Here's how the part is built. I have some questions about the finished solid (model axes, mm). A direction names the side the tool comes from. Coordinates: 2 decimals unless noted, no trailing zeros. Write each loop counter-clockwise with the first axis right and the second up, starting at its lowest first coordinate (ties: lowest second). Pieces come first, ordered by that corner, then holes. Notation, with made-up numbers: (-18.5, -9) -> (33.5, -9) arc R9 cw to (33.5, 4) -> close; hole circle Ø11 at (63.5, -28.75). An arc over 180 degrees is marked (long way). Use a Markdown table: item, result. Add a question column.
Item 1: Imagine slicing it at A-A, the plane x = 87. Write out the boundary of the cut face in (y, z).
Item 2: Will these pins go through, and if not, where does the flat tip stop? pin 1 Ø2.5 at (x, y) = (93.5, 45.5) entering from -Z; pin 2 Ø1.5 at (y, z) = (45.5, 1) entering from +X; pin 3 Ø7 at (x, y) = (-116, 28.18) entering from -Z.
Item 3: Imagine slicing it at B-B, the plane y = -3. Write out the boundary of the cut face in (x, z), and give its area (3 significant figures).
Item 4: If we mould it in two halves opening along X, with no side actions, what happens to faces 3 (the cylindrical face through (-66.77, 13.35, 1.52)), 4 (the flat face through (-134, -3, 1)), 5 (the flat face through (157, 87, 2))? For each: pulls with the +X half, pulls with the -X half, needs draft (parallel to the pull), parting line crosses it, or undercut.
Item 5: If I drill on line 1 along X through (y, z) = (32, 0.8); line 2 along Y through (x, z) = (115.25, 2.15); line 3 along Y through (x, z) = (-4, 0.8), over which ranges is the centre line in solid material (lowest first)? Write a range as from..to.
Item 6: On a 3-axis mill with a long thin cutter (end or side, diameter ignored), from which of +Z, -Z, +X, -X, +Y, -Y can I reach the whole of each face in a straight line? I mean faces 1 (the flat face through (16.99, 89.02, 1.52)), 2 (the flat face through (13, 59, 3)). Say none if no direction works.
Item 7: Imagine slicing it at C-C, the plane z = 1.2. Count the separate pieces of the cut face and the enclosed holes in it, and give its area (3 significant figures).
```python
from build123d import *

# Parameters (mm, degrees)
SKETCH1_W           = 274
SKETCH1_H           = 44
BOSS_EXTRUDE1_DEPTH = 3
SKETCH2_W           = 3
SKETCH2_H           = 25
CUT_EXTRUDE1_DEPTH  = 144.923590839
SKETCH3_W           = 274
SKETCH3_H           = 6
BOSS_EXTRUDE2_DEPTH = 3
SKETCH4_W           = 80
SKETCH4_H           = 3
CUT_EXTRUDE2_DEPTH  = 146.869804963
SKETCH6_R           = 2.1
CUT_EXTRUDE3_DEPTH  = 146.869804963
CUT_EXTRUDE4_DEPTH  = 146.869804963
SKETCH8_R           = 1.5
CUT_EXTRUDE5_DEPTH  = 3
BOSS_EXTRUDE4_DEPTH = 3
BOSS_EXTRUDE5_DEPTH = 3
FILLET2_R           = 5
BOSS_EXTRUDE6_DEPTH = 3
FILLET3_R           = 2
SKETCH13_W          = 3
SKETCH13_H          = 15
CUT_EXTRUDE6_DEPTH  = 3
CHAMFER2_SIZE       = 10
FILLET4_R           = 2
FILLET5_R           = 5
CUT_EXTRUDE9_DEPTH  = 220.631509579
FILLET6_R           = 5.5
BOSS_EXTRUDE7_DEPTH = 3
FILLET7_R           = 10
SKETCH18_R          = 4.1
CUT_EXTRUDE10_DEPTH = 220.631509579
SKETCH19_R          = 1.6
SKETCH19_W          = 3
SKETCH19_H          = 25
CUT_EXTRUDE11_DEPTH = 220.631509579
SKETCH20_R          = 3.1
CUT_EXTRUDE12_DEPTH = 220.631509579
SKETCH21_R          = 0.8
CUT_EXTRUDE13_DEPTH = 220.631509579
SKETCH22_R          = 2.1
CUT_EXTRUDE14_DEPTH = 220.631509579
SKETCH23_W          = 50
SKETCH23_H          = 25
CUT_EXTRUDE15_DEPTH = 220.631509579
FILLET8_R           = 3
SKETCH25_R          = 2.1
CUT_EXTRUDE16_DEPTH = 220.631509579


with BuildPart() as part:
    # Sketch1 → Boss-Extrude1 (new body)
    with BuildSketch(Plane.XY):
        with Locations((0, 22)):
            Rectangle(SKETCH1_W, SKETCH1_H)
    extrude(amount=BOSS_EXTRUDE1_DEPTH)

    # Sketch2 → Cut-Extrude1 (cut, through all)
    with BuildSketch(Plane.XY.offset(3)):
        with Locations((-93.5, 22)):
            Rectangle(SKETCH2_W, SKETCH2_H)
        with Locations((93.5, 22)):
            Rectangle(SKETCH2_W, SKETCH2_H)
    extrude(amount=-CUT_EXTRUDE1_DEPTH, mode=Mode.SUBTRACT)

    # Sketch3 → Boss-Extrude2 (add)
    with BuildSketch(Plane.XY.offset(3)):
        with Locations((0, 47)):
            Rectangle(SKETCH3_W, SKETCH3_H)
    extrude(amount=-BOSS_EXTRUDE2_DEPTH)

    # Sketch4 → Cut-Extrude2 (cut, through all)
    with BuildSketch(Plane.XY.offset(3)):
        with Locations((0, 45.5)):
            Rectangle(SKETCH4_W, SKETCH4_H)
    extrude(amount=-CUT_EXTRUDE2_DEPTH, mode=Mode.SUBTRACT)

    # Sketch6 → Cut-Extrude3 (cut, through all)
    with BuildSketch(Plane(origin=(0, 0, 0), x_dir=(-1, 0, 0), z_dir=(0, 0, -1))):
        with Locations((62.874847501, 21)):
            Circle(SKETCH6_R)
    extrude(amount=-CUT_EXTRUDE3_DEPTH, mode=Mode.SUBTRACT)

    # Sketch7 → Cut-Extrude4 (cut, through all)
    with BuildSketch(Plane(origin=(0, 0, 0), x_dir=(-1, 0, 0), z_dir=(0, 0, -1))):
        Polygon((0, 15), (-68.339745962, 15), (-77, 0), (0, 0), align=None)
        Polygon((68.339745962, 15), (0, 15), (0, 0), (77, 0), align=None)
    extrude(amount=-CUT_EXTRUDE4_DEPTH, mode=Mode.SUBTRACT)

    # Sketch8 → Cut-Extrude5 (cut)
    with BuildSketch(Plane(origin=(0, 0, 0), x_dir=(-1, 0, 0), z_dir=(0, 0, -1))):
        with Locations((-93.5, 45.5)):
            Circle(SKETCH8_R)
        with Locations((-115.25, 4.75)):
            Circle(SKETCH8_R)
        with Locations((-71.75, 4.75)):
            Circle(SKETCH8_R)
        with Locations((71.75, 4.75)):
            Circle(SKETCH8_R)
        with Locations(Location((115.25, 4.75, 0), (0, 0, 180))):
            Circle(SKETCH8_R)
        with Locations(Location((93.5, 45.5, 0), (0, 0, 180))):
            Circle(SKETCH8_R)
    extrude(amount=-CUT_EXTRUDE5_DEPTH, mode=Mode.SUBTRACT)

    # Sketch9 → Boss-Extrude4 (add)
    with BuildSketch(Plane(origin=(0, 0, 0), x_dir=(-1, 0, 0), z_dir=(0, 0, -1))):
        Polygon((137, 0), (122, -15), (68.339745962, -15), (68.339745962, 15), (77, 0), align=None)
    extrude(amount=-BOSS_EXTRUDE4_DEPTH)

    # Sketch10 → Boss-Extrude5 (add)
    with BuildSketch(Plane.XY.offset(3)):
        Polygon((137, 50), (137, 130), (72, 130), (72, 126.069778962), (-137, 50), align=None)
        Polygon((-51.754445725, 64), (67, 107.223083431), (67, 64), align=None, mode=Mode.SUBTRACT)
    extrude(amount=-BOSS_EXTRUDE5_DEPTH)

    # Fillet2
    fillet2_edges = [part.edges().sort_by_distance(p)[0] for p in [
        (67, 64, 1.5),
        (67, 107.223083431, 1.5),
        (-51.754445725, 64, 1.5),
    ]]
    fillet(fillet2_edges, radius=FILLET2_R)

    # Sketch11 → Boss-Extrude6 (add)
    with BuildSketch(Plane.XY.offset(3)):
        Polygon((137, 44), (154.942501021, 44), (137, 82.576377194), (137, 130), (177, 44), (177, 0), (137, 0), align=None)
    extrude(amount=-BOSS_EXTRUDE6_DEPTH)

    # Fillet3
    fillet3_edges = [part.edges().sort_by_distance(p)[0] for p in [
        (137, 44, 1.5),
        (154.942501021, 44, 1.5),
        (137, 82.576377194, 1.5),
    ]]
    fillet(fillet3_edges, radius=FILLET3_R)

    # Sketch13 → Cut-Extrude6 (cut)
    with BuildSketch(Plane.XY.offset(3)):
        with Locations((167.5, 22)):
            Rectangle(SKETCH13_W, SKETCH13_H)
    extrude(amount=-CUT_EXTRUDE6_DEPTH, mode=Mode.SUBTRACT)

    # Chamfer2
    chamfer2_edges = [part.edges().sort_by_distance(p)[0] for p in [
        (177, 0, 1.5),
    ]]
    chamfer(chamfer2_edges, length=CHAMFER2_SIZE)

    # Fillet4
    fillet4_edges = [part.edges().sort_by_distance(p)[0] for p in [
        (137, 130, 1.5),
        (72, 130, 1.5),
        (72, 126.069778962, 1.5),
        (177, 44, 1.5),
    ]]
    fillet(fillet4_edges, radius=FILLET4_R)

    # Fillet5
    fillet5_edges = [part.edges().sort_by_distance(p)[0] for p in [
        (-68.339745962, -15, 1.5),
        (-122, -15, 1.5),
        (167, 0, 1.5),
        (177, 10, 1.5),
        (77, 0, 1.5),
    ]]
    fillet(fillet5_edges, radius=FILLET5_R)

    # Sketch15 → Cut-Extrude9 (cut, through all)
    with BuildSketch(Plane(origin=(0, 0, 0), x_dir=(-1, 0, 0), z_dir=(0, 0, -1))):
        Polygon((-68.339745962, 15), (-61.411542732, 27), (54.936767243, 27), (58.339745962, 15), align=None)
    extrude(amount=-CUT_EXTRUDE9_DEPTH, mode=Mode.SUBTRACT)

    # Fillet6
    fillet6_edges = [part.edges().sort_by_distance(p)[0] for p in [
        (-58.339745962, 15, 1.5),
        (61.411542732, 27, 1.5),
        (-54.936767243, 27, 1.5),
        (-68.339745962, 15, 1.5),
    ]]
    fillet(fillet6_edges, radius=FILLET6_R)

    # Sketch17 → Boss-Extrude7 (add)
    with BuildSketch(Plane(origin=(0, 0, 0), x_dir=(-1, 0, 0), z_dir=(0, 0, -1))):
        Polygon((137, 50), (147, 46.360297657), (147, 10), (137, 0), align=None)
    extrude(amount=-BOSS_EXTRUDE7_DEPTH)

    # Fillet7
    fillet7_edges = [part.edges().sort_by_distance(p)[0] for p in [
        (-147, 10, 1.5),
        (-147, 46.360297657, 1.5),
    ]]
    fillet(fillet7_edges, radius=FILLET7_R)

    # Sketch18 → Cut-Extrude10 (cut, through all)
    with BuildSketch(Plane.XY.offset(3)):
        with Locations((87, 117)):
            Circle(SKETCH18_R)
        with Locations((127, 117)):
            Circle(SKETCH18_R)
        with Locations((87, 87.509284164)):
            Circle(SKETCH18_R)
        with Locations((127, 87.509284164)):
            Circle(SKETCH18_R)
    extrude(amount=-CUT_EXTRUDE10_DEPTH, mode=Mode.SUBTRACT)

    # Sketch19 → Cut-Extrude11 (cut, through all)
    with BuildSketch(Plane.XY.offset(3)):
        with Locations((128.5, 45.5)):
            Circle(SKETCH19_R)
        with Locations((128.5, 22)):
            Rectangle(SKETCH19_W, SKETCH19_H)
    extrude(amount=-CUT_EXTRUDE11_DEPTH, mode=Mode.SUBTRACT)

    # Sketch20 → Cut-Extrude12 (cut, through all)
    with BuildSketch(Plane(origin=(0, 0, 0), x_dir=(-1, 0, 0), z_dir=(0, 0, -1))):
        with Locations((116, 28.180148829)):
            Circle(SKETCH20_R)
    extrude(amount=-CUT_EXTRUDE12_DEPTH, mode=Mode.SUBTRACT)

    # Sketch21 → Cut-Extrude13 (cut, through all)
    with BuildSketch(Plane(origin=(0, 0, 0), x_dir=(-1, 0, 0), z_dir=(0, 0, -1))):
        with Locations((-166, 28.7)):
            Circle(SKETCH21_R)
        with Locations((-169, 15.3)):
            Circle(SKETCH21_R)
        with Locations((-166, 15.3)):
            Circle(SKETCH21_R)
        with Locations((-130, 33.7)):
            Circle(SKETCH21_R)
        with Locations((-127, 33.7)):
            Circle(SKETCH21_R)
        with Locations((-130, 10.3)):
            Circle(SKETCH21_R)
        with Locations((-127, 10.3)):
            Circle(SKETCH21_R)
        with Locations((-95, 33.7)):
            Circle(SKETCH21_R)
        with Locations((-92, 33.7)):
            Circle(SKETCH21_R)
        with Locations((-95, 10.3)):
            Circle(SKETCH21_R)
        with Locations((-92, 10.3)):
            Circle(SKETCH21_R)
        with Locations((-40, 47)):
            Circle(SKETCH21_R)
        with Locations((-40, 44)):
            Circle(SKETCH21_R)
        with Locations((40, 47)):
            Circle(SKETCH21_R)
        with Locations((40, 44)):
            Circle(SKETCH21_R)
        with Locations((95, 33.7)):
            Circle(SKETCH21_R)
        with Locations((95, 10.3)):
            Circle(SKETCH21_R)
        with Locations((-169, 28.7)):
            Circle(SKETCH21_R)
        with Locations((92, 33.7)):
            Circle(SKETCH21_R)
        with Locations((92, 10.3)):
            Circle(SKETCH21_R)
    extrude(amount=-CUT_EXTRUDE13_DEPTH, mode=Mode.SUBTRACT)

    # Sketch22 → Cut-Extrude14 (cut, through all)
    with BuildSketch(Plane(origin=(0, 0, 0), x_dir=(-1, 0, 0), z_dir=(0, 0, -1))):
        with Locations((0, 51)):
            Circle(SKETCH22_R)
        with Locations((-25, 51)):
            Circle(SKETCH22_R)
        with Locations(Location((25, 51, 0), (0, 0, 180))):
            Circle(SKETCH22_R)
    extrude(amount=-CUT_EXTRUDE14_DEPTH, mode=Mode.SUBTRACT)

    # Sketch23 → Cut-Extrude15 (cut, through all)
    with BuildSketch(Plane(origin=(0, 0, 0), x_dir=(-1, 0, 0), z_dir=(0, 0, -1))):
        with Locations((-102, 63.034014914)):
            Rectangle(SKETCH23_W, SKETCH23_H)
    extrude(amount=-CUT_EXTRUDE15_DEPTH, mode=Mode.SUBTRACT)

    # Fillet8
    fillet8_edges = [part.edges().sort_by_distance(p)[0] for p in [
        (77, 75.534014914, 1.5),
        (77, 50.534014914, 1.5),
        (127, 50.534014914, 1.5),
        (127, 75.534014914, 1.5),
    ]]
    fillet(fillet8_edges, radius=FILLET8_R)

    # Sketch25 → Cut-Extrude16 (cut, through all)
    with BuildSketch(Plane(origin=(0, 0, 0), x_dir=(-1, 0, 0), z_dir=(0, 0, -1))):
        with Locations((-67, 115.73650561)):
            Circle(SKETCH25_R)
        with Locations((-29.412295169, 102.055699877)):
            Circle(SKETCH25_R)
        with Locations((8.175409663, 88.374894144)):
            Circle(SKETCH25_R)
        with Locations((45.763114494, 74.694088411)):
            Circle(SKETCH25_R)
        with Locations((83.350819326, 61.013282678)):
            Circle(SKETCH25_R)
    extrude(amount=-CUT_EXTRUDE16_DEPTH, mode=Mode.SUBTRACT)


solid = part.part
```
Ans:
| question | item | result |
|---|---|---|
| 1 | outline | (0, 0) -> (50.53, 0) -> (50.53, 3) -> (0, 3) -> close; (75.53, 0) -> (83.41, 0) -> (83.41, 3) -> (75.53, 3) -> close; (91.61, 0) -> (112.9, 0) -> (112.9, 3) -> (91.61, 3) -> close; (121.1, 0) -> (130, 0) -> (130, 3) -> (121.1, 3) -> close |
| 2 | pin 1 | passes through |
| 2 | pin 2 | stops at x = 176.65 |
| 2 | pin 3 | stops at z = 0 |
| 3 | outline | (-134, 0) -> (-68.34, 0) -> (-68.34, 3) -> (-134, 3) -> close |
| 3 | area | 197 mm^2 |
| 4 | face 3 | undercut |
| 4 | face 4 | pulls with the -X half |
| 4 | face 5 | pulls with the +X half |
| 5 | line 1 | x = -147..-95, -92..92, 95..127, 130..177 |
| 5 | line 2 | y = 0..3.25, 6.25..50.53, 75.53..130 |
| 5 | line 3 | y = 27..44, 47..64, 81.38..98.41 |
| 6 | face 1 | +Z, -Z |
| 6 | face 2 | +Z, +X, -X, +Y, -Y |
| 7 | separate pieces | 1 |
| 7 | enclosed holes | 27 |
| 7 | area | 23,100 mm^2 |
